from build123d import *

# Parameters (mm, degrees)
F0_W      = 38.1
F0_H      = 38.1
F1_DEPTH  = 38.1
F6_DEPTH  = 38.1
F8_DEPTH  = 38.1
F9_W      = 25.4898550868
F9_H      = 7.62
F9_W_2    = 27.3198056966
F10_DEPTH = 38.1


with BuildPart() as f1:
    # F0 (on Front) → F1 (new body)
    with BuildSketch(Plane.XZ):
        with Locations((19.05, 19.05)):
            Rectangle(F0_W, F0_H)
    extrude(amount=F1_DEPTH)

    # F5 (on offset) → F6 (cut)
    with BuildSketch(Plane.YZ.offset(38.1)):
        Polygon((-11.43, 15.875), (-6.35, 38.1), (-31.75, 38.1), (-26.67, 15.875), (-21.59, 28.575), (-16.51, 28.575), align=None)
        Polygon((-25.4, 0), (-12.7, 0), (-19.05, 15.875), align=None)
        Polygon((-38.1, 0), (-31.75, 0), (-38.1, 38.1), align=None)
        Polygon((-6.35, 0), (0, 0), (0, 38.1), align=None)
    extrude(amount=-F6_DEPTH, mode=Mode.SUBTRACT)

    # F7 (on offset) → F8 (cut)
    with BuildSketch(Plane.XZ.offset(38.1)):
        Polygon((25.4, 38.1), (12.7, 38.1), (19.05, 22.225), align=None)
        Polygon((11.43, 22.225), (6.35, 0), (31.75, 0), (26.67, 22.225), (21.59, 9.525), (16.51, 9.525), align=None)
        Polygon((0, 38.1), (0, 0), (6.35, 38.1), align=None)
        Polygon((31.75, 38.1), (38.1, 0), (38.1, 38.1), align=None)
    extrude(amount=-F8_DEPTH, mode=Mode.SUBTRACT)

    # F9 (on offset) → F10 (cut)
    with BuildSketch(Plane.XY.offset(38.1)):
        with Locations((25.3550724566, -11.43)):
            Rectangle(F9_W, F9_H)
        with Locations((13.6599028483, -26.67)):
            Rectangle(F9_W_2, F9_H)
    extrude(amount=-F10_DEPTH, mode=Mode.SUBTRACT)


solid = f1.part
Part model, mm, in its own coordinate system. A direction names the side the tool comes from. Coordinates: 2 decimals unless noted, no trailing zeros. Loops run counter-clockwise (first coordinate to the right, second up) from the corner with the lowest first, then second, coordinate; pieces in that order, holes last. Notation, with made-up numbers: M 65,58 L 77,58 A11 cw 77,63 Z; hole C 46,44.5 d8. An arc over 180 degrees is marked long. Use a Markdown table: item, result. Add a question column.
Q1. Mould opens along Y. For faces 5 (the flat face through (19.32, -3.13, 19.32)), 6 (the flat face through (3.13, -9.05, 18.78)), 7 (the flat face through (28, -19, 28.575)) say: +Y half, -Y half, draft (parallel to the pull), parting line (faces both ways), or undercut.
Q2. Probe L1, parallel to Y at x = 21, z = 15.5; L2, parallel to Y at x = 8.5, z = 16.5; L3, parallel to Y at x = 9, z = 25.5. List the from-to ranges inside material, lowest first.
Q3. Which spindle directions (+Z, -Z, +X, -X, +Y, -Y) get a long thin tool onto all of the face, cutting with end or side? Do faces 1 (the flat face through (5.06, -15.83, 7.83)), 2 (the flat face through (8.87, -8.926, 26.832)), 3 (the flat face through (12.61, -8, 23)), 4 (the flat face through (24.166, -32.449, 15.964)). Say none if no direction does.
Q4. Cut at C-C (x = 21). Give the number of separate pieces and of enclosed holes in the cut face, and give its area (3 significant figures).
Q5. Pin check, flat tips, straight feed: P1, Ø5.5, axis at x = 15.5, z = 13, coming from the -Y side (3 decimals); P2, Ø6, axis at y = -29, z = 27, coming from the +X side; P3, Ø2.5, axis at y = -29.5, z = 27, coming from the -X side. Stop position of each tip, or through.
Q6. Cut at B-B (z = 27.5). Write the cut outline in (x, y).
Q7. Cut at A-A (z = 34). Write the cut outline in (x, y), and give its area (3 significant figures).
Worked out:
| question | item | result |
|---|---|---|
| 1 | face 5 | +Y half |
| 1 | face 6 | draft |
| 1 | face 7 | undercut |
| 2 | L1 | y = -34.33 to -30.48, -22.86 to -19.2, -18.9 to -15.24, -7.62 to -3.77 |
| 2 | L2 | y = -34.5 to -30.48, -22.86 to -11.68, -11.29 to -3.6 |
| 2 | L3 | y = -36 to -30.48, -22.82 to -15.28, -9.23 to -2.1 |
| 3 | face 1 | -Z, +X, -X |
| 3 | face 2 | +Z, +X, -X |
| 3 | face 3 | +Z, -Z, +X |
| 3 | face 4 | -Z, +Y, -Y |
| 4 | separate pieces | 3 |
| 4 | enclosed holes | 0 |
| 4 | area | 269 mm2 |
| 5 | P1 | stops at y = -34.375 |
| 5 | P2 | stops at x = 34.1 |
| 5 | P3 | stops at x = 4.37 |
| 6 | outline | M 4.58,-36.33 L 16.94,-36.33 L 16.94,-30.48 L 4.58,-30.48 Z; M 4.58,-22.02 L 16.94,-22.02 L 16.94,-16.08 L 4.58,-16.08 Z; M 4.58,-8.77 L 12.61,-8.77 L 12.61,-7.62 L 16.94,-7.62 L 16.94,-1.77 L 4.58,-1.77 Z; M 21.16,-36.33 L 33.52,-36.33 L 33.52,-29.33 L 27.32,-29.33 L 27.32,-30.48 L 21.16,-30.48 Z; M 21.16,-22.02 L 33.52,-22.02 L 33.52,-16.08 L 21.16,-16.08 Z; M 21.16,-7.62 L 33.52,-7.62 L 33.52,-1.77 L 21.16,-1.77 Z |
| 7 | outline | M 5.67,-37.42 L 14.34,-37.42 L 14.34,-30.81 L 5.67,-30.81 Z; M 5.67,-7.29 L 14.34,-7.29 L 14.34,-0.68 L 5.67,-0.68 Z; M 23.76,-37.42 L 32.43,-37.42 L 32.43,-30.81 L 23.76,-30.81 Z; M 23.76,-7.29 L 32.43,-7.29 L 32.43,-0.68 L 23.76,-0.68 Z |
| 7 | area | 229 mm2 |
